from build123d import *

# Parameters (mm, degrees)
SKETCH1_W           = 44
SKETCH1_H           = 20
BOSS_EXTRUDE1_DEPTH = 26
SKETCH3_W           = 44
SKETCH3_H           = 5.5
BOSS_EXTRUDE5_DEPTH = 2.5
SKETCH2_R           = 2.8
CUT_EXTRUDE1_DEPTH  = 29.5
SKETCH4_R           = 5
CUT_EXTRUDE2_DEPTH  = 21
SKETCH5_W           = 8
SKETCH5_H           = 4.5
CUT_EXTRUDE3_DEPTH  = 21
SKETCH6_W           = 10
SKETCH6_H           = 5.5
CUT_EXTRUDE4_DEPTH  = 2.5


with BuildPart() as part:
    # Sketch1 → Boss-Extrude1 (new body)
    with BuildSketch(Plane(origin=(0, 0, 0), x_dir=(1, 0, 0), z_dir=(0, 1, 0))):
        with Locations((21.30324178, 10)):
            Rectangle(SKETCH1_W, SKETCH1_H)
    extrude(amount=BOSS_EXTRUDE1_DEPTH)

    # Sketch3 → Boss-Extrude5 (add)
    with BuildSketch(Plane.XZ):
        with Locations((21.30324178, -10)):
            Rectangle(SKETCH3_W, SKETCH3_H)
    extrude(amount=BOSS_EXTRUDE5_DEPTH)

    # Sketch2 → Cut-Extrude1 (cut, through all)
    with BuildSketch(Plane(origin=(0, 26, 0), x_dir=(1, 0, 0), z_dir=(0, 1, 0))):
        with Locations((8.80324178, 10)):
            Circle(SKETCH2_R)
        with Locations((33.80324178, 10)):
            Circle(SKETCH2_R)
        with Locations((21.30324178, 10)):
            Circle(SKETCH2_R)
    extrude(amount=-CUT_EXTRUDE1_DEPTH, mode=Mode.SUBTRACT)

    # Sketch4 → Cut-Extrude2 (cut)
    with BuildSketch(Plane(origin=(0, 26, 0), x_dir=(1, 0, 0), z_dir=(0, 1, 0))):
        with Locations((21.30324178, 10)):
            Circle(SKETCH4_R)
    extrude(amount=-CUT_EXTRUDE2_DEPTH, mode=Mode.SUBTRACT)

    # Sketch5 → Cut-Extrude3 (cut, through all)
    with BuildSketch(Plane(origin=(0, 0, -20), x_dir=(-1, 0, 0), z_dir=(0, 0, -1))):
        with Locations((-33.80324178, 13.75)):
            Rectangle(SKETCH5_W, SKETCH5_H)
        with Locations((-8.80324178, 13.75)):
            Rectangle(SKETCH5_W, SKETCH5_H)
    extrude(amount=-CUT_EXTRUDE3_DEPTH, mode=Mode.SUBTRACT)

    # Sketch6 → Cut-Extrude4 (cut)
    with BuildSketch(Plane.XZ.offset(2.5)):
        with Locations((21.30324178, -10)):
            Rectangle(SKETCH6_W, SKETCH6_H)
    extrude(amount=-CUT_EXTRUDE4_DEPTH, mode=Mode.SUBTRACT)


solid = part.part
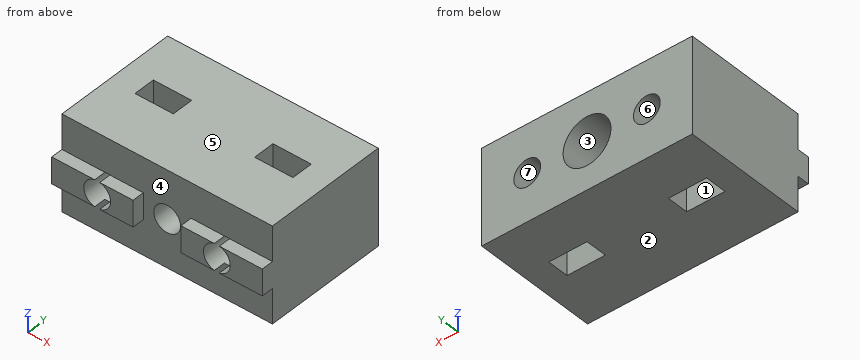
Verification items for the finished model (mm, model axes). Face numbers are marked on the shaded views. A direction names the side the tool comes from. Round coordinates to 2 decimals unless told otherwise and drop trailing zeros. Loops run counter-clockwise (first coordinate to the right, second up) from the corner with the lowest first, then second, coordinate; pieces in that order, holes last. Notation, with made-up numbers: M -36,13 L -31,13 A25 cw -31,48 Z; hole C 74.25,-26.5 d10. An arc over 180 degrees is marked long. Write each question's results on one line, items separated by ' | '.
1) Scan lines: L1, parallel to X at y = 19.5, z = -10; L2, parallel to X at y = 12.75, z = -10; L3, parallel to X at y = 13.75, z = -18.25. Record each from-to range of solid material in increasing order. Write a range as from..to.
Checks:
L1: x = -0.7..6, 11.6..16.3, 26.3..31, 36.6..43.3 | L2: x = -0.7..4.8, 12.8..16.3, 26.3..29.8, 37.8..43.3 | L3: x = -0.7..4.8, 12.8..29.8, 37.8..43.3
2) Gauge pin test, flat ends, axial feed: P1, Ø2, axis at x = 5, y = -1.5, coming from the +Z side; P2, Ø9, axis at x = 21.3, z = -10, coming from the +Y side. Record the tip position at first contact, or that the pin passes through.
Checks:
P1: stops at z = -7.25 | P2: stops at y = 5
3) Section check A-A on y = 6. Record the boundary of the cut face in (x, z), then the cut area to 3 significant figures.
Checks:
outline: M -0.7,-20 L 43.3,-20 L 43.3,0 L -0.7,0 Z; hole C 8.8,-10 d5.6; hole C 21.3,-10 d10; hole C 33.8,-10 d5.6 | area: 752 mm2
4) Mould release check, pull along Z, two halves, no side actions. Record for the marked faces 4, 5, 6 and 7: released by +Z, released by -Z, zero draft, split by the parting line, or undercut.
Checks:
face 4: zero draft | face 5: released by +Z | face 6: undercut | face 7: undercut
5) Section check C-C on x = 13.5. Record the boundary of the cut face in (y, z).
Checks:
outline: M -2.5,-12.75 L 0,-12.75 L 0,-20 L 26,-20 L 26,0 L 0,0 L 0,-7.25 L -2.5,-7.25 Z
6) Access from +Z, -Z, +X, -X, +Y, -Y to the whole of each face (thin tool, end or side, straight path). Record for the marked faces 1, 2 and 3.
Checks:
face 1: +Z, -Z | face 2: -Z, +X, -X, +Y, -Y | face 3: +Y
7) Section check B-B on z = -4. Record the boundary of the cut face in (x, y).
Checks:
outline: M -0.7,0 L 43.3,0 L 43.3,26 L -0.7,26 Z; hole M 4.8,11.5 L 12.8,11.5 L 12.8,16 L 4.8,16 Z; hole M 29.8,11.5 L 37.8,11.5 L 37.8,16 L 29.8,16 Z
8) Section check D-D on y = 0.5. Record the boundary of the cut face in (x, z).
Checks:
outline: M -0.7,-20 L 43.3,-20 L 43.3,0 L -0.7,0 Z; hole C 8.8,-10 d5.6; hole C 21.3,-10 d5.6; hole C 33.8,-10 d5.6
